The listing builds one solid part. Answer for the finished solid, in the listing's coordinates (mm). Face numbers are marked on the shaded views. Coordinates: 2 decimals unless noted, no trailing zeros. Order: outer loops, then holes, each group sorted by start corner. A loop starts at its lowest first (then second) coordinate and runs counter-clockwise, first axis right, second up. Notation, with made-up numbers: (34.5, 86) -> (68.5, 86) arc R21 ccw to (68.5, 112) -> close; hole circle Ø1 at (12, 70). An arc over 180 degrees is marked (long way). Answer in a Markdown table with one row per item.
Autodesk Inventor part; units mm, degrees
ref_plane "YZ Plane" through (0, 0, 0) normal (1, 0, 0) x (0, 1, 0)
ref_plane "XZ Plane" through (0, 0, 0) normal (0, 1, 0) x (-1, 0, 0)
ref_plane "XY Plane" through (0, 0, 0) normal (0, 0, 1) x (1, 0, 0)
sketch "スケッチ1" plane through (0, 0, 0) normal (0, 1, 0) x (1, 0, 0)
  circle A0 centre (0, 0) radius 2.5
  circle A1 centre (0, 0) radius 1.3
  dimension "d0" = 5
  dimension "d1" = 2.6
extrude "押し出し1" add sketch "スケッチ1" along normal mid plane 8
chamfer "面取り1" distance 0.2 angle 45 2 edges at (-2.5, 4, 0) (-2.5, -4, 0)
properties part number "ARL-2608E"
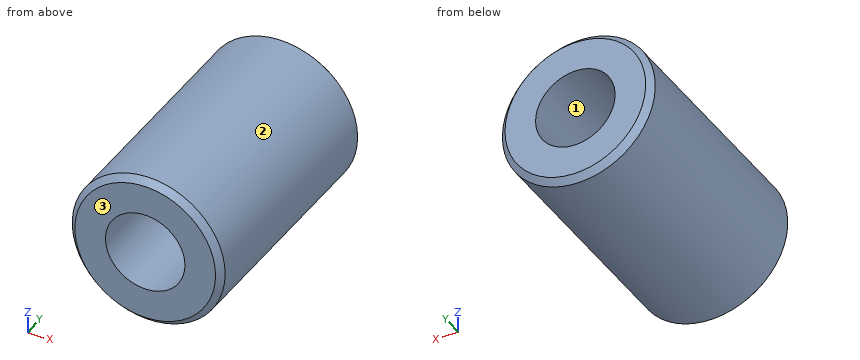
(1) A flat-ended cylindrical pin translates along its axis: pin 1 (1.5 mm diameter, centred on x = 1.5, y = -1, fed in from +Z). Find the tip coordinate at first contact, or state that the pin passes through.
Check values:
| item | result |
|---|---|
| pin 1 | z = 2.38 |
(2) Find the intervals of material crossed by line 1 along X through (y, z) = (0, 0); line 2 along Z through (x, y) = (-1.15, 3.5), in increasing order. Write a range as from..to.
Check values:
| item | result |
|---|---|
| line 1 | -2.5..-1.3, 1.3..2.5 |
| line 2 | -2.22..-0.61, 0.61..2.22 |
(3) A cutting plane is placed at B-B, the plane z = 0. Determine the outline of the cut face in (x, y).
Check values:
| item | result |
|---|---|
| outline | (-2.5, -3.8) -> (-2.3, -4) -> (-1.3, -4) -> (-1.3, 4) -> (-2.3, 4) -> (-2.5, 3.8) -> close; (1.3, -4) -> (2.3, -4) -> (2.5, -3.8) -> (2.5, 3.8) -> (2.3, 4) -> (1.3, 4) -> close |
(4) A cutting plane is placed at A-A, the plane x = 0. Determine the outline of the cut face in (y, z).
Check values:
| item | result |
|---|---|
| outline | (-4, -2.3) -> (-3.8, -2.5) -> (3.8, -2.5) -> (4, -2.3) -> (4, -1.3) -> (-4, -1.3) -> close; (-4, 1.3) -> (4, 1.3) -> (4, 2.3) -> (3.8, 2.5) -> (-3.8, 2.5) -> (-4, 2.3) -> close |
(5) A cutting plane is placed at C-C, the plane y = 3.25. Determine the outline of the cut face in (x, z), then the cut area to 3 significant figures.
Check values:
| item | result |
|---|---|
| outline | circle Ø5 at (0, 0); hole circle Ø2.6 at (0, 0) |
| area | 14.3 mm² |
(6) For a pull along Z with two mould halves and no side action, classify the marked faces 1, 2 and 3 as released by +Z, released by -Z, zero draft, split by the parting line, or undercut.
Check values:
| item | result |
|---|---|
| face 1 | undercut |
| face 2 | split by the parting line |
| face 3 | zero draft |
